Part model, mm, in its own coordinate system. Face numbers are marked on the shaded views. A direction names the side the tool comes from. Coordinates: 2 decimals unless noted, no trailing zeros. Write each loop counter-clockwise with the first axis right and the second up, starting at its lowest first coordinate (ties: lowest second). Pieces come first, ordered by that corner, then holes. Notation, with made-up numbers: (69.25, 26) -> (121.25, 26) arc R12 ccw to (121.25, 36) -> close; hole circle Ø11 at (84, 21). An arc over 180 degrees is marked (long way). Write item = value, one per line. Start each with the question number.
Q1. Pin check, flat tips, straight feed: P1, Ø3, axis at x = 0.5, y = 2, coming from the +Z side; P2, Ø1.1, axis at y = 2, z = -1, coming from the +X side. Stop position of each tip, or through.
Q2. Probe line 1 (Y direction, x = 0, z = -2.45); line 2 (X direction, y = 0, z = -0.7); line 3 (X direction, y = -1.25, z = -2.25). List the from-to ranges inside material, lowest first.
Q3. Band-saw the part on A-A, the plane y = 0. List the corners of the cut face in (x, z), plus the area to 3 significant figures.
Q4. Band-saw the part on B-B, the plane z = -3.35. List the corners of the cut face in (x, y).
Q5. Band-saw the part on D-D, the plane y = -2.25. List the corners of the cut face in (x, z).
Q6. Band-saw the part on C-C, the plane x = 0. List the corners of the cut face in (y, z).
Q7. Tool access for the marked faces 1 and 2: list every direction of +Z, -Z, +X, -X, +Y, -Y with a clear straight run to the whole face (end or side of a thin tool).
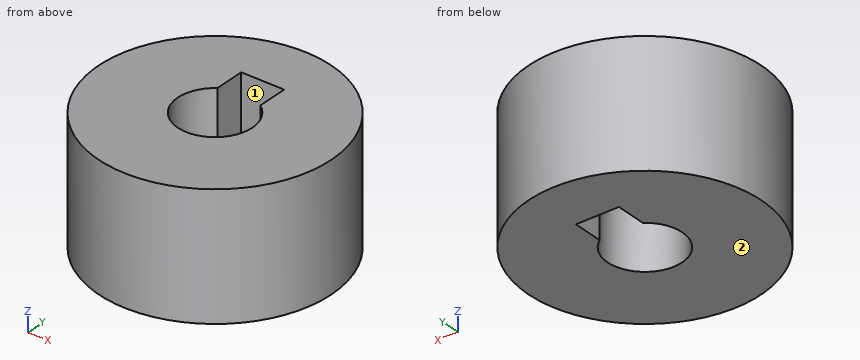
from build123d import *

# Parameters (mm, degrees)
SKETCH1_W           = 3.5
SKETCH1_H           = 3
CUT_EXTRUDE2_DEPTH  = 4
SKETCH7_R           = 5.15
BOSS_EXTRUDE3_DEPTH = 2.5


with BuildPart() as part:
    # Sketch1 → Revolve1 (revolve)
    with BuildSketch(Plane(origin=(0, 0, 0), x_dir=(1, 0, 0), z_dir=(0, 1, 0))):
        with Locations((3.4, 3.069926874)):
            Rectangle(SKETCH1_W, SKETCH1_H)
    revolve(axis=Axis((0, 0, 0), (0, 0, -1)))

    # Sketch6 → Cut-Extrude2 (cut)
    with BuildSketch(Plane.XY.offset(-1.569926874)):
        with BuildLine():
            Line((-0.95, 2.7), (-0.95, 1.349073756))
            ThreePointArc((-0.95, 1.349073756), (0, 1.65), (0.95, 1.349073756))
            Line((0.95, 1.349073756), (0.95, 2.7))
            Line((0.95, 2.7), (-0.95, 2.7))
        make_face()
    extrude(amount=-CUT_EXTRUDE2_DEPTH, mode=Mode.SUBTRACT)

    # Sketch7 → Boss-Extrude3 (add)
    with BuildSketch(Plane.XY.offset(-1.569926874)):
        Circle(SKETCH7_R)
        with BuildLine():
            Line((0.95, 2.7), (0.95, 1.349073756))
            ThreePointArc((0.95, 1.349073756), (0, -1.65), (-0.95, 1.349073756))
            Line((-0.95, 1.349073756), (-0.95, 2.7))
            Line((-0.95, 2.7), (0.95, 2.7))
        make_face(mode=Mode.SUBTRACT)
    extrude(amount=BOSS_EXTRUDE3_DEPTH)


solid = part.part
Ans:
q1.P1 = 0.93
q1.P2 = 4.94
q2.line_1 = -5.15 to -1.65, 2.7 to 5.15
q2.line_2 = -5.15 to -1.65, 1.65 to 5.15
q2.line_3 = -5 to -1.08, 1.08 to 5
q3.outline = (-5.15, -4.57) -> (-1.65, -4.57) -> (-1.65, 0.93) -> (-5.15, 0.93) -> close; (1.65, -4.57) -> (5.15, -4.57) -> (5.15, 0.93) -> (1.65, 0.93) -> close
q3.area = 38.5 mm2
q4.outline = circle Ø10.3 at (0, 0); hole (-0.95, 1.35) arc R1.65 ccw (long way) to (0.95, 1.35) -> (0.95, 2.7) -> (-0.95, 2.7) -> close
q5.outline = (-4.63, -4.57) -> (4.63, -4.57) -> (4.63, 0.93) -> (-4.63, 0.93) -> close
q6.outline = (-5.15, -4.57) -> (-1.65, -4.57) -> (-1.65, 0.93) -> (-5.15, 0.93) -> close; (2.7, -4.57) -> (5.15, -4.57) -> (5.15, 0.93) -> (2.7, 0.93) -> close
q7.face_1 = +Z, -Z
q7.face_2 = -Z, +X, -X, +Y, -Y
